Autodesk Inventor part; units mm, degrees
ref_plane "YZ Plane" through (0, 0, 0) normal (1, 0, 0) x (0, 1, 0)
ref_plane "XZ Plane" through (0, 0, 0) normal (0, 1, 0) x (-1, 0, 0)
ref_plane "XY Plane" through (0, 0, 0) normal (0, 0, 1) x (1, 0, 0)
sketch "Sketch1" plane through (0, 0, 0) normal (1, 0, 0) x (0, 1, 0)
  line L0 (0, 0) -> (76.2, 0)
  line L1 (76.2, 0) -> (76.2, -3.175)
  line L2 (76.2, -3.175) -> (0, -3.175)
  line L3 (0, -3.175) -> (0, 0)
  line L4 (76.2, 0) -> (73.025, 0)
  line L5 (73.025, 0) -> (73.025, -25.4)
  line L6 (73.025, -25.4) -> (76.2, -25.4)
  line L7 (76.2, -25.4) -> (76.2, 0)
  dimension "d0" = 76.2
  dimension "d1" = 3.175
  dimension "d2" = 3.175
  dimension "d3" = 25.4
extrude "Extrusion1" add sketch "Sketch1" along normal blind 92.6846
sketch "Sketch2" plane through (0, 76.2, 0) normal (0, 1, 0) x (1, 0, 0)
  line L0 (0, 0) -> (92.6846, 0)
  line L1 (0, 25.4) -> (0, 0)
  line L2 (46.3423, -68.8852) -> (46.3423, 85.7759) construction
  point P0 (4.5466, 7.7216)
  point P1 (40.4622, 7.7216)
  point P2 (88.138, 7.7216)
  point P3 (52.2224, 7.7216)
  dimension "d6" = 7.7216
  dimension "d7" = 4.5466
  dimension "d8" = 0
  dimension "d9" = 35.9156
  dimension "d27" = 92.6846
  dimension "d28" = 46.3423
hole "Hole1" at (4.5466, 76.2, -7.7216) at (40.4622, 76.2, -7.7216) at (88.138, 76.2, -7.7216) at (52.2224, 76.2, -7.7216) direction (0, -1, 0) diameter 4.9784 depth 25.4 tip angle 118
sketch "Sketch3" plane through (0, 76.2, 0) normal (0, 1, 0) x (1, 0, 0)
  circle A0 centre (22.5044, 25.6794) radius 14.2875 construction
  circle A1 centre (40.4622, 7.7216) radius 2.4892 construction
  point P0 (0, 0)
  dimension "d17" = 28.575
  dimension "d18" = 17.9578
  dimension "d19" = 17.9578
hole "Hole2" at (22.5044, 76.2, -25.6794) direction (0, -1, 0) diameter 31.75 depth 25.4 tip angle 118
sketch "Sketch4" plane through (0, 76.2, 0) normal (0, 1, 0) x (1, 0, 0)
  circle A0 centre (88.138, 7.7216) radius 2.4892
  point P0 (0, 0)
  point P1 (70.1802, 25.6794)
  dimension "d29" = 17.9578
  dimension "d30" = 17.9578
hole "Hole3" at (70.1802, 76.2, -25.6794) direction (0, -1, 0) diameter 19.05 depth 25.4 tip angle 118
sketch "Sketch5" plane through (0, 0, -3.175) normal (0, 0, -1) x (-1, 0, 0)
  line L0 (0, 0) -> (-92.6846, 0)
  line L1 (-92.6846, 0) -> (-92.6846, 73.025)
  line L2 (0, 0) -> (0, 73.025)
  line L3 (0, 73.025) -> (-6.6319, 73.025)
  line L4 (-79.7011, 73.025) -> (-92.6846, 73.025)
  point P0 (-79.9846, 47.625)
  point P1 (-12.7, 47.625)
  point P2 (-12.7, 12.7)
  point P3 (-79.9846, 12.7)
  dimension "d38" = 12.7
  dimension "d39" = 12.7
  dimension "d40" = 12.7
  dimension "d41" = 12.7
  dimension "d42" = 12.7
  dimension "d43" = 25.4
  dimension "d44" = 25.4
  dimension "d45" = 12.7
hole "Hole4" at (79.9846, 47.625, -3.175) at (12.7, 47.625, -3.175) at (12.7, 12.7, -3.175) at (79.9846, 12.7, -3.175) direction (0, 0, 1) diameter 4.4958 end through all countersink diameter 8.4328 countersink angle 82
equation "\"d28\" = 0.5 * d27"
properties part number "CAR_044_180VersaLBracketMount" material "Aluminum 6061"
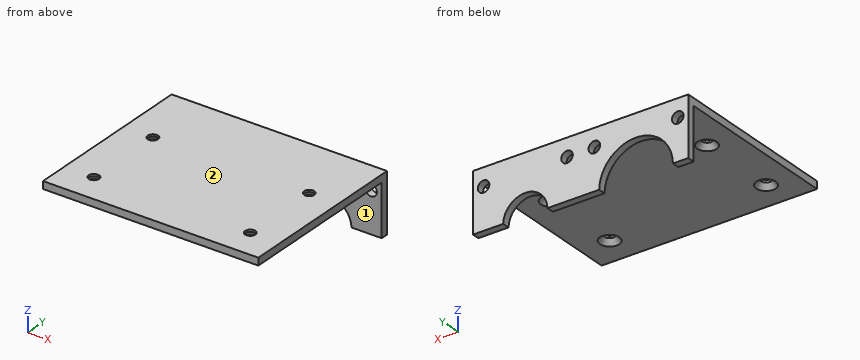
Work out the finished part from the listing and answer in its coordinate system (mm). Face numbers are marked on the shaded views. A direction names the side the tool comes from. Round coordinates to 2 decimals unless told otherwise and drop trailing zeros. Order: outer loops, then holes, each group sorted by start corner. A loop starts at its lowest first (then second) coordinate and runs counter-clockwise, first axis right, second up.
Q1. A cutting plane is placed at B-B, the plane x = 12.7. Determine the outline of the cut face in (y, z) (1 decimal).
Solution:
outline: (0, -3.2) - (8.5, -3.2) - (10.5, -0.9) - (10.5, 0) - (0, 0) - close; (14.9, -0.9) - (16.9, -3.2) - (43.4, -3.2) - (45.4, -0.9) - (45.4, 0) - (14.9, 0) - close; (49.9, -0.9) - (51.8, -3.2) - (73, -3.2) - (73, -13.2) - (76.2, -13.2) - (76.2, 0) - (49.9, 0) - close
Q2. A cutting plane is placed at D-D, the plane x = 45.5. Determine the outline of the cut face in (y, z) (3 decimals), then the cut area to 4 significant figures.
Solution:
outline: (0, -3.175) - (73.025, -3.175) - (73.025, -25.4) - (76.2, -25.4) - (76.2, 0) - (0, 0) - close
area: 312.5 mm2
Q3. A cutting plane is placed at C-C, the plane z = -23.5. Determine the outline of the cut face in (x, y) (3 decimals).
Solution:
outline: (0, 73.025) - (6.78, 73.025) - (6.78, 76.2) - (0, 76.2) - close; (38.229, 73.025) - (60.908, 73.025) - (60.908, 76.2) - (38.229, 76.2) - close; (79.453, 73.025) - (92.685, 73.025) - (92.685, 76.2) - (79.453, 76.2) - close
Q4. Find the intervals of material crossed by line 1 along X through (y, z) = (12.7, -0.65); line 2 along Y through (x, z) = (82.5, -2.25); line 3 along Z through (x, y) = (19, 31) (3 decimals), in increasing order.
Solution:
line 1: x = 0 to 10.45, 14.95 to 77.74, 82.23 to 92.68
line 2: y = 0 to 10.39, 15.01 to 45.32, 49.93 to 76.2
line 3: z = -3.175 to 0
Q5. A tool of negligible diameter and unlimited length cuts with its end or side. For the marked faces 1 and 2, from which of +Z, -Z, +X, -X, +Y, -Y can it reach the whole face along a straight path? Write none if from no direction.
Solution:
face 1: -Z, +X, -X, -Y
face 2: +Z, +X, -X, +Y, -Y
Q6. A cutting plane is placed at A-A, the plane y = 12.7. Determine the outline of the cut face in (x, z) (1 decimal).
Solution:
outline: (0, -3.2) - (8.5, -3.2) - (10.5, -0.9) - (10.5, 0) - (0, 0) - close; (14.9, -0.9) - (16.9, -3.2) - (75.8, -3.2) - (77.7, -0.9) - (77.7, 0) - (14.9, 0) - close; (82.2, -0.9) - (84.2, -3.2) - (92.7, -3.2) - (92.7, 0) - (82.2, 0) - close
Q7. Given pin 1 Ø3.5 at (x, y) = (79.98, 12.7) entering from -Z; pin 2 Ø6.5 at (x, z) = (88.14, -7.72) entering from +Y; pin 3 Ø6 at (x, z) = (83.5, -10) entering from -Y (3 decimals); pin 4 Ø3 at (x, y) = (62.5, 39) entering from -Z (3 decimals), each flat-ended and moving along its own axis, determine where each tip first touches the part or whether it passes through.
Solution:
pin 1: passes through
pin 2: stops at y = 76.2
pin 3: stops at y = 73.025
pin 4: stops at z = -3.175
